from build123d import *

# Parameters (mm, degrees)
F1_DEPTH = 25
F0_R     = 3
F2_DEPTH = 25


# Not quite as in the source:
# - ends of sketch curves that miss each other by under 0.0002 mm in the source are joined


with BuildPart() as f1:
    # F0 (on Front) → F1 (new body)
    with BuildSketch(Plane.XZ):
        with BuildLine():
            ThreePointArc((-35.5724336391, 25.151316084), (-36.2194536929, 21.8985163721), (-38.0620115133, 19.1409229296))
            Line((-38.0620115133, 19.1409229296), (-40.551597873, 16.6513245695))
            Line((-40.551597873, 16.6513245695), (-42.4208999514, 14.7820134806))
            ThreePointArc((-42.4208999514, 14.7820134806), (-39.3014754977, 15.797816289), (-36.6477945425, 17.7267127756))
            ThreePointArc((-36.6477945425, 17.7267127756), (-34.0584132659, 28.3087511137), (-42.2491526952, 35.491801885))
            ThreePointArc((-42.2491526952, 35.491801885), (-43.1573109451, 35.6113615168), (-44.0724336391, 35.651316084))
            Line((-44.0724336391, 35.651316084), (-44.0724336391, 33.651316084))
            ThreePointArc((-44.0724336391, 33.651316084), (-43.3316200297, 33.6189719105), (-42.5964443036, 33.5221855419))
            ThreePointArc((-42.5964443036, 33.5221855419), (-37.5610624566, 30.6150186129), (-35.5724336391, 25.151316084))
        make_face()
    extrude(amount=F1_DEPTH)

    # F0 (on Front) → F2 (join)
    with BuildSketch(Plane.XZ):
        with BuildLine():
            Line((-44.0724072079, 15.3363250258), (-44.0724107491, 16.651316084))
            ThreePointArc((-44.0724107491, 16.651316084), (-52.5724336391, 25.151304639), (-44.0724336391, 33.651316084))
            Line((-44.0724336391, 33.651316084), (-44.0724336391, 35.651316084))
            Line((-44.0724336391, 35.651316084), (-44.0724336391, 40.651316084))
            Line((-44.0724336391, 40.651316084), (-58.0724336391, 40.651316084))
            Line((-58.0724336391, 40.651316084), (-58.0722360097, 19.007240245))
            Line((-58.0722360097, 19.007240245), (-47.893068168, 13.1304188771))
            Line((-47.893068168, 13.1304188771), (-44.0724072079, 15.3363250258))
        make_face()
        Polygon((-18.7646776515, 35.6099158673), (-36.6477945425, 17.7267127756), (-41.2439775428, 13.1305076206), (-26.2214527658, -1.8919447448), (-18.7646776515, -9.348683916), (-9.0724336391, -9.348683916), (-9.0724336391, 35.6099158673), align=None)
        with Locations((-21.2439775428, 1.1096808038)):
            Circle(F0_R, mode=Mode.SUBTRACT)
        with Locations((-31.2439775428, 13.1305076206)):
            Circle(F0_R, mode=Mode.SUBTRACT)
        with Locations((-21.2439775428, 25.1513302219)):
            Circle(F0_R, mode=Mode.SUBTRACT)
        with BuildLine():
            ThreePointArc((-42.2491526952, 35.491801885), (-34.0584132659, 28.3087511137), (-36.6477945425, 17.7267127756))
            Line((-36.6477945425, 17.7267127756), (-18.7646776515, 35.6099158673))
            Line((-18.7646776515, 35.6099158673), (-9.0724336391, 35.6099158673))
            Line((-9.0724336391, 35.6099158673), (-9.0724336391, 40.651316084))
            Line((-9.0724336391, 40.651316084), (-18.7646776515, 40.651316084))
            Line((-18.7646776515, 40.651316084), (-44.0724336391, 40.651316084))
            Line((-44.0724336391, 40.651316084), (-44.0724336391, 35.651316084))
            ThreePointArc((-44.0724336391, 35.651316084), (-43.1573109451, 35.6113615168), (-42.2491526952, 35.491801885))
        make_face()
        with BuildLine():
            Line((-44.0723953274, 10.9245988987), (-47.893068168, 13.1304188771))
            Line((-47.893068168, 13.1304188771), (-58.0721286869, 7.2534116208))
            Line((-58.0721286869, 7.2534116208), (-58.0719770953, -9.348683916))
            Line((-58.0719770953, -9.348683916), (-21.593111593, -9.348683916))
            Line((-21.593111593, -9.348683916), (-27.6356629198, -3.3061617156))
            Line((-27.6356629198, -3.3061617156), (-29.3171299504, -1.62470279))
            Line((-29.3171299504, -1.62470279), (-38.061976782, 7.1201018897))
            ThreePointArc((-38.061976782, 7.1201018897), (-36.2193967899, 4.3624994422), (-35.5723688964, 1.1096808038))
            ThreePointArc((-35.5723688964, 1.1096808038), (-50.0827684437, -4.9007349291), (-44.0723917864, 9.6096808038))
            Line((-44.0723917864, 9.6096808038), (-44.0723953274, 10.9245988987))
        make_face()
        Polygon((-58.0721286869, 7.2534116208), (-47.893068168, 13.1304188771), (-58.0722360097, 19.007240245), align=None)
        Polygon((-18.7646776515, -9.348683916), (-26.2214527658, -1.8919447448), (-27.6356629198, -3.3061617156), (-21.593111593, -9.348683916), align=None)
    extrude(amount=F2_DEPTH)


solid = f1.part
The listing builds one solid part. Answer for the finished solid, in the listing's coordinates (mm). A direction names the side the tool comes from. Round coordinates to 2 decimals unless told otherwise and drop trailing zeros. Loops run counter-clockwise (first coordinate to the right, second up) from the corner with the lowest first, then second, coordinate; pieces in that order, holes last. Notation, with made-up numbers: M -9,-24 L 29,-24 A30 ccw 29,9 Z; hole C 20,-16 d8. An arc over 180 degrees is marked long. Return JSON: item names as keys, results as strings.
Q1. Find section B-B, the plane x = -27. Determine the outline of the cut face in (y, z), plus the area to 3 significant figures.
Results list:
{"outline": "M -25,-9.35 L 0,-9.35 L 0,-2.67 L -25,-2.67 Z; M -25,-1.11 L 0,-1.11 L 0,40.65 L -25,40.65 Z", "area": "1,210 mm2"}
Q2. The mould has two halves that part along X. Classify faces 1 (the face through (-34, -12, -9.349)), 2 (the face through (-33.455, -12.325, 15.158)), 3 (the face through (-9.072, -12, 15)): released by +X, released by -X, zero draft, split by the parting line, or undercut.
Results list:
{"face 1": "zero draft", "face 2": "undercut", "face 3": "released by +X"}
Q3. Find section D-D, the plane x = -33. Determine the outline of the cut face in (y, z), plus the area to 3 significant figures.
Results list:
{"outline": "M -25,-9.35 L 0,-9.35 L 0,2.06 L -25,2.06 Z; M -25,4.89 L 0,4.89 L 0,10.7 L -25,10.7 Z; M -25,15.56 L 0,15.56 L 0,40.65 L -25,40.65 Z", "area": "1,060 mm2"}
Q4. Find section C-C, the plane y = -15.5. Determine the outline of the cut face in (x, z), plus the area to 3 significant figures.
Results list:
{"outline": "M -58.07,-9.35 L -9.07,-9.35 L -9.07,40.65 L -58.07,40.65 Z; hole M -47.89,13.13 L -44.07,10.92 L -44.07,9.61 A8.5 ccw long -35.57,1.11 A8.5 ccw -38.06,7.12 L -27.64,-3.31 L -26.22,-1.89 L -41.24,13.13 L -36.65,17.73 A10.5 cw -42.42,14.78 L -38.06,19.14 A8.5 ccw long -44.07,16.65 L -44.07,15.34 Z; hole C -31.24,13.13 d6; hole C -21.24,1.11 d6; hole C -21.24,25.15 d6", "area": "1,840 mm2"}
Q5. Find the intervals of material crossed by line 1 along Z through (x, y) = (-21, -13.25); line 2 along Z through (x, y) = (-22.5, -17.25); line 3 along X through (y, z) = (-8.25, 12), in increasing order. Write a range as from..to.
Results list:
{"line 1": "z = -9.35..-1.88, 4.1..22.16, 28.14..40.65", "line 2": "z = -9.35..-1.61, 3.83..22.43, 27.88..40.65", "line 3": "x = -58.07..-45.94, -40.11..-34.02, -28.47..-9.07"}
Q6. Find section A-A, the plane z = 8.5. Determine the outline of the cut face in (x, y).
Results list:
{"outline": "M -58.07,-25 L -48.27,-25 L -48.27,0 L -58.07,0 Z; M -36.61,-25 L -9.07,-25 L -9.07,0 L -36.61,0 Z"}
Q7. Which of the six approach directions +Z, -Z, +X, -X, +Y, -Y give full straight-line access (tool end or side, diameter ignored) to faces 4 (the face through (-46.009, -12.325, 14.218)), 5 (the face through (-33, -12, 40.651))?
Results list:
{"face 4": "+Y, -Y", "face 5": "+Z, +X, -X, +Y, -Y"}
